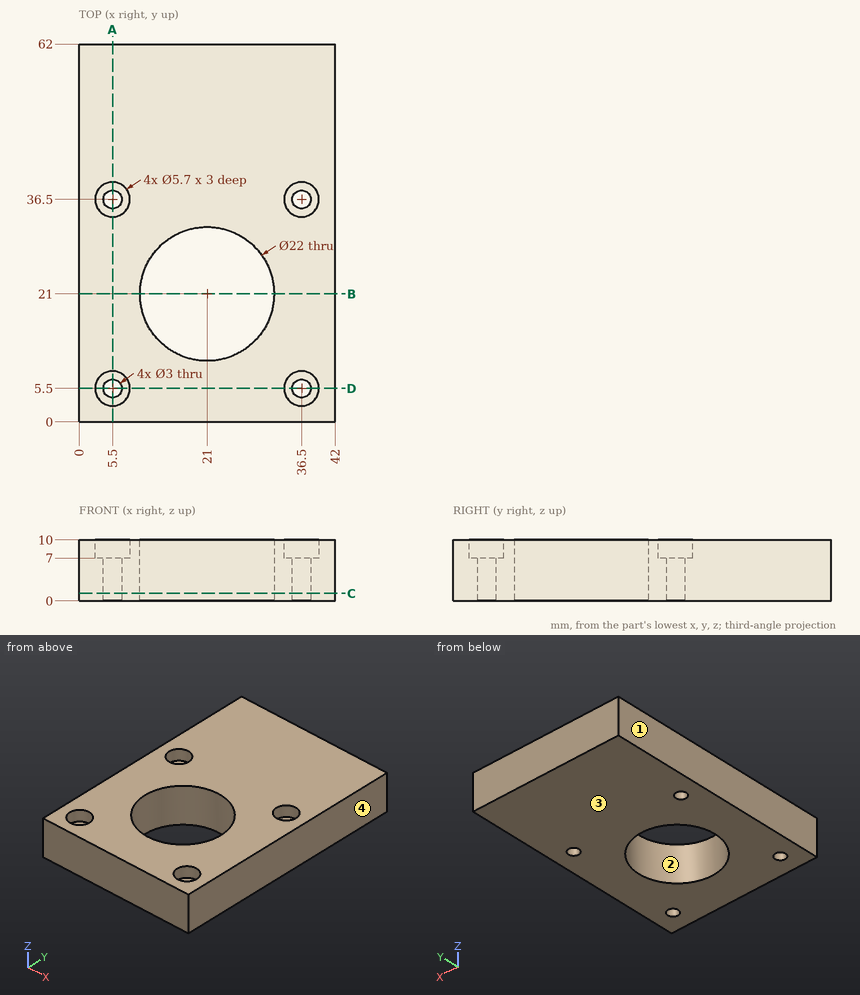
Geometry: see drawing. Coordinates: mm, zero at the bounding-box minimum. Round coordinates to 2 decimals unless told otherwise and drop trailing zeros. Order: outer loops, then holes, each group sorted by start corner. A loop starts at its lowest first (then second) coordinate and runs counter-clockwise, first axis right, second up. Notation, with made-up numbers: (37, 7) - (91, 7) arc R11 cw to (91, 23) - close; hole circle Ø1 at (-35, -40). An arc over 180 degrees is marked (long way). Use a Markdown table: item, result. Add a question column.
1. Section query D-D (y = 5.5). Return the cut outline in (x, z), then the cut area to 3 significant figures.
2. Section query A-A (x = 5.5). Return the cut outline in (y, z), then the cut area to 3 significant figures.
3. Section query B-B (y = 21). Return the cut outline in (x, z).
4. Line query: probe 1 along Y at (x, z) = (5.5, 2.25); probe 2 along Y at (x, z) = (36.5, 9); probe 3 along Z at (x, y) = (35.5, 4). Output: solid intervals per line, ascending.
5. Section query C-C (z = 1.25). Return the cut outline in (x, y), then the cut area to 3 significant figures.
6. Mould query, pull axis X, two halves, no side actions, for the marked faces 1, 2, 3 and 4. Classes: +X half, -X half, draft (parallel to the pull), parting line (faces both ways), or undercut.
7. First-contact query: pin 1 (3 mm diameter, centred on x = 36.5, y = 6.5, fed in from +Z); pin 2 (6 mm diameter, centred on y = 52.5, z = 2, fed in from -X); pin 3 (20 mm diameter, centred on x = 21, y = 21, fed in from -Z). Flat tips, straight axial feed; report the tip coordinate or a pass-through.
Derived:
| question | item | result |
|---|---|---|
| 1 | outline | (0, 0) - (4, 0) - (4, 7) - (2.65, 7) - (2.65, 10) - (0, 10) - close; (7, 0) - (35, 0) - (35, 7) - (33.65, 7) - (33.65, 10) - (8.35, 10) - (8.35, 7) - (7, 7) - close; (38, 0) - (42, 0) - (42, 10) - (39.35, 10) - (39.35, 7) - (38, 7) - close |
| 1 | area | 344 mm2 |
| 2 | outline | (0, 0) - (4, 0) - (4, 7) - (2.65, 7) - (2.65, 10) - (0, 10) - close; (7, 0) - (35, 0) - (35, 7) - (33.65, 7) - (33.65, 10) - (8.35, 10) - (8.35, 7) - (7, 7) - close; (38, 0) - (62, 0) - (62, 10) - (39.35, 10) - (39.35, 7) - (38, 7) - close |
| 2 | area | 544 mm2 |
| 3 | outline | (0, 0) - (10, 0) - (10, 10) - (0, 10) - close; (32, 0) - (42, 0) - (42, 10) - (32, 10) - close |
| 4 | probe 1 | 0 to 4, 7 to 35, 38 to 62 |
| 4 | probe 2 | 0 to 2.65, 8.35 to 33.65, 39.35 to 62 |
| 4 | probe 3 | 0 to 7 |
| 5 | outline | (0, 0) - (42, 0) - (42, 62) - (0, 62) - close; hole circle Ø3 at (5.5, 5.5); hole circle Ø3 at (5.5, 36.5); hole circle Ø22 at (21, 21); hole circle Ø3 at (36.5, 5.5); hole circle Ø3 at (36.5, 36.5) |
| 5 | area | 2,200 mm2 |
| 6 | face 1 | -X half |
| 6 | face 2 | undercut |
| 6 | face 3 | draft |
| 6 | face 4 | +X half |
| 7 | pin 1 | z = 7 |
| 7 | pin 2 | x = 0 |
| 7 | pin 3 | through |
